```python
from build123d import *

# Parameters (mm, degrees)
SKETCH1_R           = 9.5
BOSS_EXTRUDE1_DEPTH = 10
SKETCH2_W           = 50.0481005
SKETCH2_H           = 5
CUT_EXTRUDE1_DEPTH  = 10


with BuildPart() as part:
    # Sketch1 → Boss-Extrude1 (new body)
    with BuildSketch(Plane.XY):
        with BuildLine():
            Line((-25, -20), (25, -20))
            add(Edge.make_bspline(
                [(18.732474137, -7.006740519), (19.213565223, -16.256662958), (25, -20)],
                knots=[0, 0, 0, 0.763362407, 0.763362407, 0.763362407], degree=2))
            ThreePointArc((18.732474137, -7.006740519), (0, 20), (-18.732474137, -7.006740519))
            add(Edge.make_bspline(
                [(-18.732474137, -7.006740519), (-19.393359213, -16.636844777), (-25, -20)],
                knots=[0, 0, 0, 0.631911459, 0.631911459, 0.631911459], degree=2))
        make_face()
        Circle(SKETCH1_R, mode=Mode.SUBTRACT)
    extrude(amount=BOSS_EXTRUDE1_DEPTH)

    # Sketch2 → Cut-Extrude1 (cut)
    with BuildSketch(Plane.XY.offset(10)):
        with Locations((0.02405025, -17.5)):
            Rectangle(SKETCH2_W, SKETCH2_H)
    extrude(amount=-CUT_EXTRUDE1_DEPTH, mode=Mode.SUBTRACT)


solid = part.part
```
Geometry: final body of the model. Coordinates: model frame, mm. Round coordinates to 2 decimals unless told otherwise and drop trailing zeros. Write each loop counter-clockwise with the first axis right and the second up, starting at its lowest first coordinate (ties: lowest second). Pieces come first, ordered by that corner, then holes. Notation, with made-up numbers: (20, 55) -> (59, 55) arc R18 ccw to (59, 60) -> close; hole circle Ø9 at (-10.75, 86.5). An arc over 180 degrees is marked (long way). Return JSON: item names as keys, results as strings.
Q1. Section B-B on y = 0. Return the cut outline in (x, z).
From the geometry:
{"outline": "(-20, 0) -> (-9.5, 0) -> (-9.5, 10) -> (-20, 10) -> close; (9.5, 0) -> (20, 0) -> (20, 10) -> (9.5, 10) -> close"}
Q2. First-contact query: pin 1 Ø6 at (x, z) = (-5.5, 4.5) entering from +Y; pin 2 Ø1.5 at (y, z) = (-5, 3.5) entering from -X; pin 3 Ø1 at (y, z) = (-1.5, 3) entering from -X (3 decimals). Flat tips, straight axial feed; report the tip coordinate or a pass-through.
From the geometry:
{"pin 1": "y = 19.84", "pin 2": "x = -19.54", "pin 3": "x = -19.975"}
Q3. Mould query, pull axis Y, two halves, no side actions, for faces 1 (the flat face through (-9.4, 2.7, 10)), 2 (the cylindrical face through (4.38, -8.43, 4.93)), 3 (the flat face through (0, -15, 5)). Classes: +Y half, -Y half, draft (parallel to the pull), parting line (faces both ways), or undercut.
From the geometry:
{"face 1": "draft", "face 2": "undercut", "face 3": "-Y half"}
Q4. Section A-A on x = 0. Return the cut outline in (y, z), and give its area (3 significant figures).
From the geometry:
{"outline": "(-15, 0) -> (-9.5, 0) -> (-9.5, 10) -> (-15, 10) -> close; (9.5, 0) -> (20, 0) -> (20, 10) -> (9.5, 10) -> close", "area": "160 mm2"}
Q5. Ray query, line 1 (Y direction, x = 0, z = 6); line 2 (Y direction, x = 7.5, z = 5.75); line 3 (X direction, y = 6, z = 1). Return the intervals inside material, ascending.
From the geometry:
{"line 1": "-15 to -9.5, 9.5 to 20", "line 2": "-15 to -5.83, 5.83 to 18.54", "line 3": "-19.08 to -7.37, 7.37 to 19.08"}
Q6. Section C-C on x = 16. Return the cut outline in (y, z), and give its area (3 significant figures).
From the geometry:
{"outline": "(-15, 0) -> (12, 0) -> (12, 10) -> (-15, 10) -> close", "area": "270 mm2"}
Q7. Section D-D on y = 13. Return the cut outline in (x, z).
From the geometry:
{"outline": "(-15.2, 0) -> (15.2, 0) -> (15.2, 10) -> (-15.2, 10) -> close"}
